For this review, use the dimensioned drawing (mm, ordinates from the lowest corner) and the shaded views. A direction names the side the tool comes from. Round coordinates to 2 decimals unless told otherwise and drop trailing zeros. Order: outer loops, then holes, each group sorted by start corner. A loop starts at its lowest first (then second) coordinate and runs counter-clockwise, first axis right, second up. Notation, with made-up numbers: (-29.75, 13) - (25.25, 13) arc R17 ccw to (25.25, 40) - close; hole circle Ø5 at (43, 30.25). An arc over 180 degrees is marked (long way). Write item = value, one per line.
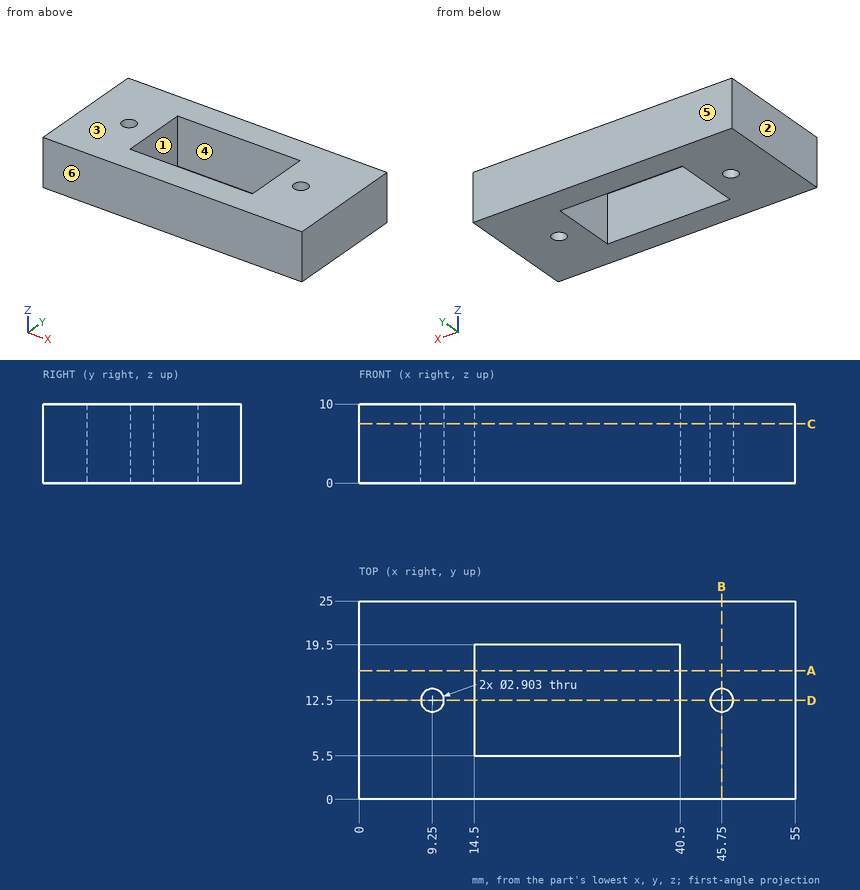
1) Clearance check with a flat-ended pin moving along its axis: pin 1 Ø1 at (x, y) = (38.5, 10.5) entering from -Z. State where the tip first meets the part, or that it passes through.
Findings:
pin_1 = through
2) We need section A-A on y = 16.25. Write out the cut boundary in (x, z), and give its area (3 significant figures).
Findings:
outline = (0, 0) - (14.5, 0) - (14.5, 10) - (0, 10) - close; (40.5, 0) - (55, 0) - (55, 10) - (40.5, 10) - close
area = 290 mm^2
3) The part is to be moulded in two halves that separate along Y. For the marked faces 3, 4, 5 and 6, say which applies: released by +Y, released by -Y, zero draft, split by the parting line, or undercut.
Findings:
face_3 = zero draft
face_4 = undercut
face_5 = released by +Y
face_6 = released by -Y
4) We need section D-D on y = 12.5. Write out the cut boundary in (x, z), and give its area (3 significant figures).
Findings:
outline = (0, 0) - (7.8, 0) - (7.8, 10) - (0, 10) - close; (10.7, 0) - (14.5, 0) - (14.5, 10) - (10.7, 10) - close; (40.5, 0) - (44.3, 0) - (44.3, 10) - (40.5, 10) - close; (47.2, 0) - (55, 0) - (55, 10) - (47.2, 10) - close
area = 232 mm^2
5) We need section C-C on z = 7.5. Write out the cut boundary in (x, y), and give its area (3 significant figures).
Findings:
outline = (0, 0) - (55, 0) - (55, 25) - (0, 25) - close; hole circle Ø2.9 at (9.25, 12.5); hole (14.5, 5.5) - (40.5, 5.5) - (40.5, 19.5) - (14.5, 19.5) - close; hole circle Ø2.9 at (45.75, 12.5)
area = 998 mm^2
6) We need section B-B on x = 45.75. Write out the cut boundary in (y, z).
Findings:
outline = (0, 0) - (11.05, 0) - (11.05, 10) - (0, 10) - close; (13.95, 0) - (25, 0) - (25, 10) - (13.95, 10) - close
7) For the marked faces 1 and 2, list the 3-axis set-ups (+Z, -Z, +X, -X, +Y, -Y) from which the entire face can be reached by the end or side of a thin tool; tool diameter is ignored.
Findings:
face_1 = +Z, -Z
face_2 = +Z, -Z, -X, +Y, -Y
8) To check wall thickness, follow L1, parallel to X at y = 8, z = 6.75; L2, parallel to Y at x = 9.25, z = 6; L3, parallel to Y at x = 23, z = 1.5. State the ranges of each line that lie inside material, in increasing order. Write a range as from..to.
Findings:
L1 = 0..14.5, 40.5..55
L2 = 0..11.05, 13.95..25
L3 = 0..5.5, 19.5..25
